Source: CAD feature listing. Evaluate the final solid. Frame: model axes, mm. A direction names the side the tool comes from. Give positions to 0.01 mm unless a question says otherwise; leave off trailing zeros. Order: outer loops, then holes, each group sorted by start corner. A loop starts at its lowest first (then second) coordinate and runs counter-clockwise, first axis right, second up.
```python
from build123d import *

# Parameters (mm, degrees)
F0_W     = 38.1
F0_H     = 10.4394
F1_DEPTH = 13.97
F2_T     = -2.54
F4_D     = 8.89
F4_DEPTH = 2.54


with BuildPart() as f1:
    # F0 (on Top) → F1 (new body)
    with BuildSketch(Plane.XY):
        Rectangle(F0_W, F0_H)
    extrude(amount=F1_DEPTH)

    # F2
    f2_openings = [f1.faces().sort_by_distance(p)[0] for p in [
        (0, 0, 13.97),
    ]]
    offset(amount=F2_T, openings=f2_openings)

    # F4
    with Locations(Plane.XZ.offset(5.2197)):
        with Locations((-8.89, 6.985), (8.89, 6.985)):
            Hole(F4_D / 2, depth=F4_DEPTH)


solid = f1.part
```
1) Reachability of faces 1 (the flat face through (0, -5.22, 7)), 2 (the cylindrical face through (-5.363, -3.932, 4.28)), 3 (the flat face through (0, 2.68, 8)) from +Z, -Z, +X, -X, +Y, -Y: full face, straight path, thin tool, end or side. Return the list, or none.
Report:
face 1: +Z, -Z, +X, -X, -Y
face 2: -Y
face 3: +Z
2) Material intervals for L1, parallel to Y at x = -5, z = 13; L2, parallel to Z at x = -8.89, y = -4.1; L3, parallel to X at y = -0.25, z = 6, sorted ascending.
Report:
L1: y = -5.22 to -2.68, 2.68 to 5.22
L2: z = 0 to 2.54, 11.43 to 13.97
L3: x = -19.05 to -16.51, 16.51 to 19.05
3) Draft query along X for faces 4 (the flat face through (-19.05, 0, 7)), 5 (the flat face through (0, 0, 2.54)), 6 (the flat face through (0, 4, 13.97)). Return one class per face: +X half, -X half, draft (parallel to the pull), parting line (faces both ways), or undercut.
Report:
face 4: -X half
face 5: undercut
face 6: draft
4) Section query B-B, the plane x = -11. Return the cut outline in (y, z), and give its area (3 significant figures).
Report:
outline: (-5.22, 0) - (5.22, 0) - (5.22, 13.97) - (2.68, 13.97) - (2.68, 2.54) - (-2.68, 2.54) - (-2.68, 3.07) - (-5.22, 3.07) - close; (-5.22, 10.9) - (-2.68, 10.9) - (-2.68, 13.97) - (-5.22, 13.97) - close
area: 64.7 mm2
5) Pin query (flat end, axial travel): pin 1 (4.5 mm diameter, centred on x = 1, y = 0, fed in from +Z); pin 2 (5.5 mm diameter, centred on x = -8.89, z = 6.985, fed in from -Y). Return the tip coordinate at first contact, or that it passes through.
Report:
pin 1: stops at z = 2.54
pin 2: stops at y = 2.68
6) Section query A-A, the plane z = 9.75. Return the cut outline in (x, y), and give its area (3 significant figures).
Report:
outline: (-19.05, -5.22) - (-12.37, -5.22) - (-12.37, -2.68) - (-16.51, -2.68) - (-16.51, 2.68) - (16.51, 2.68) - (16.51, -2.68) - (12.37, -2.68) - (12.37, -5.22) - (19.05, -5.22) - (19.05, 5.22) - (-19.05, 5.22) - close; (-5.41, -5.22) - (5.41, -5.22) - (5.41, -2.68) - (-5.41, -2.68) - close
area: 185 mm2
7) Section query C-C, the plane y = 0.75. Return the cut outline in (x, z), and give its area (3 significant figures).
Report:
outline: (-19.05, 0) - (19.05, 0) - (19.05, 13.97) - (16.51, 13.97) - (16.51, 2.54) - (-16.51, 2.54) - (-16.51, 13.97) - (-19.05, 13.97) - close
area: 155 mm2
8) Section query D-D, the plane x = -15. Return the cut outline in (y, z).
Report:
outline: (-5.22, 0) - (5.22, 0) - (5.22, 13.97) - (2.68, 13.97) - (2.68, 2.54) - (-2.68, 2.54) - (-2.68, 13.97) - (-5.22, 13.97) - close
